```python
from build123d import *

# Parameters (mm, degrees)
SKETCH1_W           = 38.1
SKETCH1_H           = 93.875
BOSS_EXTRUDE1_DEPTH = 3.175
SKETCH2_W           = 6.35
SKETCH2_H           = 3.175
CUT_EXTRUDE1_DEPTH  = 102.361759308
FILLET1_R           = 2.54


with BuildPart() as part:
    # Sketch1 → Boss-Extrude1 (new body)
    with BuildSketch(Plane(origin=(0, 0, 0), x_dir=(1, 0, 0), z_dir=(0, 1, 0))):
        with Locations((19.05, 46.9375)):
            Rectangle(SKETCH1_W, SKETCH1_H)
    extrude(amount=BOSS_EXTRUDE1_DEPTH)

    # Sketch2 → Cut-Extrude1 (cut, through all)
    with BuildSketch(Plane(origin=(0, 3.175, 0), x_dir=(1, 0, 0), z_dir=(0, 1, 0))):
        with Locations((9.525, 85.9375)):
            Rectangle(SKETCH2_W, SKETCH2_H)
        with Locations((28.575, 85.9375)):
            Rectangle(SKETCH2_W, SKETCH2_H)
    extrude(amount=-CUT_EXTRUDE1_DEPTH, mode=Mode.SUBTRACT)

    # Fillet1
    fillet1_edges = [part.edges().sort_by_distance(p)[0] for p in [
        (0, 1.5875, -93.875),
        (38.1, 1.5875, -93.875),
        (38.1, 1.5875, 0),
        (0, 1.5875, 0),
    ]]
    fillet(fillet1_edges, radius=FILLET1_R)


solid = part.part
```
The model under review builds one solid part; all positions refer to its coordinate system, in mm. A direction names the side the tool comes from. Round coordinates to 2 decimals unless told otherwise and drop trailing zeros. Loops run counter-clockwise (first coordinate to the right, second up) from the corner with the lowest first, then second, coordinate; pieces in that order, holes last.
1) Clearance check with a flat-ended pin moving along its axis: P1, Ø3, axis at x = 12, z = -73, coming from the -Y side. State where the tip first meets the part, or that it passes through.
Values follow:
P1: stops at y = 0
2) Wall thickness on line 1 along Z through (x, y) = (27.5, 0.5) (3 decimals); line 2 along Z through (x, y) = (36.5, 2.65): over which ranges is each line inside the solid? List them lowest first.
Values follow:
line 1: z = -93.875 to -87.525, -84.35 to 0
line 2: z = -93.69 to -0.18
3) Consider section A-A on x = 28. State the section outline as (y, z) points (3 decimals).
Values follow:
outline: (0, -93.875) - (3.175, -93.875) - (3.175, -87.525) - (0, -87.525) - close; (0, -84.35) - (3.175, -84.35) - (3.175, 0) - (0, 0) - close
4) The part is to be moulded in two halves that separate along X. For faces 1 (the face through (37.336, 1.61, -0.724)), 2 (the face through (31.75, 2, -86)), 3 (the face through (19, 3.175, -48)), say which applies: pulls with the +X half, pulls with the -X half, needs draft (parallel to the pull), parting line crosses it, or undercut.
Values follow:
face 1: pulls with the +X half
face 2: undercut
face 3: needs draft
5) Tool access review of faces 4 (the face through (25.4, 2, -86)), 5 (the face through (0, 2, -46)): name each direction out of +Z, -Z, +X, -X, +Y, -Y from which nothing blocks a thin tool from reaching the whole face with its end or side.
Values follow:
face 4: +Y, -Y
face 5: +Z, -Z, -X, +Y, -Y
